```python
from build123d import *

# Parameters (mm, degrees)
SKETCH1_R             = 9.813093158
BOSS_EXTRUDE1_DEPTH   = 10
SKETCH1_R_2           = 10.498292465
BOSS_EXTRUDE1_2_DEPTH = 10
BOSS_EXTRUDE1_3_DEPTH = 10
SKETCH2_R             = 52.823312211
BOSS_EXTRUDE2_DEPTH   = 10


with BuildPart() as part:
    # Sketch1 → Boss-Extrude1 (new body)
    with BuildSketch(Plane(origin=(0, 0, 0), x_dir=(1, 0, 0), z_dir=(0, 1, 0))):
        with Locations(Location((-31.119938379, 20.059237389, 0), (0, 0, 270))):
            Circle(SKETCH1_R)
    extrude(amount=BOSS_EXTRUDE1_DEPTH)



with BuildPart() as body_2:
    # Sketch1 → Boss-Extrude1 2 (new body)
    with BuildSketch(Plane(origin=(0, 0, 0), x_dir=(1, 0, 0), z_dir=(0, 1, 0))):
        with Locations(Location((19.335746107, 20.059237389, 0), (0, 0, 270))):
            Circle(SKETCH1_R_2)
    extrude(amount=BOSS_EXTRUDE1_2_DEPTH)


with BuildPart() as body_3:
    # Sketch1 → Boss-Extrude1 3 (new body)
    with BuildSketch(Plane(origin=(0, 0, 0), x_dir=(1, 0, 0), z_dir=(0, 1, 0))):
        with BuildLine():
            ThreePointArc((-37.654984417, -21.345137195), (-7.123841316, -33.991550742), (23.407301786, -21.345137195))
            ThreePointArc((23.407301786, -21.345137195), (23.407301786, -14.274069383), (16.336233974, -14.274069383))
            ThreePointArc((16.336233974, -14.274069383), (-7.123841316, -23.991550742), (-30.583916606, -14.274069383))
            ThreePointArc((-30.583916606, -14.274069383), (-37.654984417, -14.274069383), (-37.654984417, -21.345137195))
        make_face()
    extrude(amount=BOSS_EXTRUDE1_3_DEPTH)


with BuildPart() as part_1:
    add(part.part)

    add(body_2.part)  # Boss-Extrude2 merges body 2

    add(body_3.part)  # Boss-Extrude2 merges body 3
    # Sketch2 → Boss-Extrude2 (add)
    with BuildSketch(Plane.XZ):
        with Locations(Location((-6.251130616, -4.246879691, 0), (0, 0, 270))):
            Circle(SKETCH2_R)
    extrude(amount=BOSS_EXTRUDE2_DEPTH)


solid = part_1.part
```
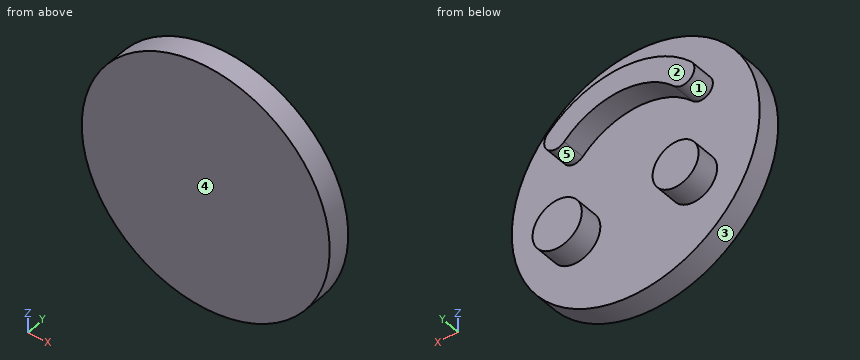
Read the model definition and answer for the solid it produces. Units are mm, in the model's axes. Face numbers are marked on the shaded views. A direction names the side the tool comes from. Give positions to 0.01 mm unless a question says otherwise; leave off trailing zeros. Loops run counter-clockwise (first coordinate to the right, second up) from the corner with the lowest first, then second, coordinate; pieces in that order, holes last.
Item 1: The mould has two halves that part along X. Classify the marked faces 3, 4 and 5: released by +X, released by -X, zero draft, split by the parting line, or undercut.
Item 2: The part is cut by section B-B (x = -11). Write down the section's boundary in (y, z).
Item 3: The part is cut by section C-C (z = -24). Write down the section's boundary in (x, y).
Item 4: Each of these flat-tipped pins is pushed along its axis until it touches: pin 1 Ø2 at (x, y) = (7, -6) entering from +Z; pin 2 Ø6 at (y, z) = (7, 26.5) entering from +X; pin 3 Ø6 at (x, y) = (9.5, -1.5) entering from +Z. Where does it stop, or does it pass through?
Item 5: For the marked faces 1 and 2, determine the directions among +Z, -Z, +X, -X, +Y, -Y from which every point of the face is accessible in a straight line to the end or side of a thin tool.
Item 6: The part is cut by section D-D (y = -7.25). Write down the section's boundary in (x, z).
Item 7: The part is cut by section A-A (y = 3.5). Write down the section's boundary in (x, z), and give its area (3 significant figures).
Item 8: Find the intervals of material crossed by line 1 along X through (y, z) = (5.25, -20.5); line 2 along Y through (x, z) = (10, -35.5); line 3 along X through (y, z) = (2, -24), in increasing order.
Taken from the geometry:
1. face 3: split by the parting line
1. face 4: zero draft
1. face 5: undercut
2. outline: (-10, -56.86) - (0, -56.86) - (0, 23.76) - (10, 23.76) - (10, 33.82) - (0, 33.82) - (0, 48.36) - (-10, 48.36) - close
3. outline: (-55.24, -10) - (42.74, -10) - (42.74, 0) - (29.07, 0) - (29.07, 10) - (9.61, 10) - (9.61, 0) - (-22.13, 0) - (-22.13, 10) - (-40.11, 10) - (-40.11, 0) - (-55.24, 0) - close
4. pin 1: stops at z = 47.14
4. pin 2: stops at x = 21.09
4. pin 3: stops at z = 47.01
5. face 1: +Y
5. face 2: +Z, -Z, +X, -X, +Y
6. outline: circle Ø105.65 at (-6.25, -4.25)
7. outline: circle Ø19.63 at (-31.12, -20.06); (-37.65, 21.35) arc R5 ccw to (-30.58, 14.27) arc R33.18 cw to (16.34, 14.27) arc R5 ccw to (23.41, 21.35) arc R43.18 ccw to start; circle Ø21 at (19.34, -20.06)
7. area: 1,330 mm2
8. line 1: x = -40.92 to -21.32, 8.85 to 29.82
8. line 2: y = -10 to 0
8. line 3: x = -40.11 to -22.13, 9.61 to 29.07
